Input: part model. Units: mm. Frame: model coordinates. A direction names the side the tool comes from. Give positions to 0.01 mm unless a question says otherwise; leave off trailing zeros. Loops run counter-clockwise (first coordinate to the right, second up) from the corner with the lowest first, then second, coordinate; pieces in that order, holes last. Notation, with made-up numbers: (51, 0) -> (63, 0) arc R7 cw to (63, 9) -> close; hole circle Ø5 at (18, 33). An arc over 180 degrees is marked (long way). One line per question, with ' | ' between items.
Autodesk Inventor part; units mm, degrees
ref_plane "YZ Plane" through (0, 0, 0) normal (1, 0, 0) x (0, 1, 0)
ref_plane "XZ Plane" through (0, 0, 0) normal (0, 1, 0) x (-1, 0, 0)
ref_plane "XY Plane" through (0, 0, 0) normal (0, 0, 1) x (1, 0, 0)
sketch "Sketch1" plane through (0, 0, 0) normal (1, 0, 0) x (0, 1, 0)
  arc A0 (-67.3092, -213.4776) -> (57.9334, -216.2104) centre (0, 0) ccw
  arc A1 (-69.6961, -221.0477) -> (59.9878, -223.8775) centre (0, 0) ccw construction
  line L0 (0, 0) -> (-69.6961, -221.0477) construction
  line L1 (0, 0) -> (59.9878, -223.8775) construction
  line L2 (59.9878, -223.8775) -> (57.9334, -216.2104) construction
  line L3 (0, -287.3347) -> (0, 47.8891) construction
  arc A2 (-69.6961, -227.6971) -> (59.9878, -230.4452) centre (0, 0) ccw
  arc A3 (-68.5027, -217.2627) -> (58.9606, -220.0439) centre (0, 0) ccw construction
  arc A4 (-68.5027, -217.2627) -> (-53.1803, -221.5119) centre (0, 0) ccw
  line L4 (-53.1803, -221.5119) -> (0, 0) construction
  arc A5 (-35.1466, -206.5815) -> (27.3518, -207.7573) centre (0, 0) ccw construction
  line L5 (0, 0) -> (27.3518, -207.7573) construction
  line L6 (0, 0) -> (209.55, 0) construction
  circle A6 centre (27.3518, -207.7573) radius 15.5575
  circle A7 centre (-35.1466, -206.5815) radius 15.5575
  line L7 (59.9878, -230.4452) -> (57.9334, -216.2104)
  line L8 (-69.6961, -227.6971) -> (-67.3092, -213.4776)
  point P0 (-26.7758, -226.2272)
  point P1 (0, -227.8063)
  point P2 (26.7758, -226.2272)
  point P3 (53.1803, -221.5119)
  point P4 (35.5128, -221.0024)
  point P5 (22.8969, -222.6633)
  point P6 (-31.2556, -221.6446)
  point P7 (-43.8, -219.5103)
  dimension "d0" = 223.8375
  dimension "d1" = 231.775
  dimension "d2" = 32.5
  dimension "d3" = 15
  dimension "d4" = 238.125
  dimension "d5" = 4
  dimension "d8" = 27
  dimension "d19" = 209.55
  dimension "d20" = 82.5
  dimension "d21" = 62.5094
  dimension "d22" = 31.115
  dimension "d23" = 31.115
extrude "Extrusion1" add sketch "Sketch1" along normal blind 2.54 contours A0 A7 A6 L7 A2 L8
hole "Hole1" at (0, -53.1803, -221.5119) at (0, -26.7758, -226.2272) at (0, 0, -227.8063) at (0, 26.7758, -226.2272) at (0, 53.1803, -221.5119) direction (1, 0, 0) diameter 3.2004 end through all
fillet "Fillet1" radius 3.175 8 edges at (1.27, 57.9334, -216.2104) (1.27, 59.9878, -230.4452) (1.27, 35.5128, -221.0024) (1.27, 22.8969, -222.6633) (1.27, -31.2556, -221.6446) (1.27, -43.8, -219.5103) (1.27, -67.3092, -213.4776) (1.27, -69.6961, -227.6971)
properties part number "3DPRINT,HOOD,ALIGNMENT,PLATES" material "Nylon 6/6"
1. Pin query (flat end, axial travel): P1, Ø2.5, axis at y = -26.78, z = -226.23, coming from the -X side; P2, Ø1.5, axis at x = 1.5, z = -219.5, coming from the +Y side. Return the tip coordinate at first contact, or that it passes through.
Determined:
P1: passes through | P2: stops at y = 58.52
2. Ray query, line 1 along Z through (x, y) = (0.85, 0) (1 decimal); line 2 along Z through (x, y) = (1.45, 25.5); line 3 along Z through (x, y) = (0.55, 34.5). Return the intervals inside material, ascending. Write a range as from..to.
Determined:
line 1: z = -238.1..-229.4, -226.2..-223.8 | line 2: z = -236.76..-227.19, -225.26..-223.2 | line 3: z = -235.61..-221.58
3. Section query B-B (x = 1.7). Count the separate pieces of the cut face and the enclosed holes in it, then the cut area to 3 significant figures.
Determined:
separate pieces: 1 | enclosed holes: 5 | area: 1,770 mm2
4. Section query D-D (y = -42). Output: boundary loops of the cut face in (x, z), then the cut area to 3 significant figures.
Determined:
outline: (0, -234.39) -> (2.54, -234.39) -> (2.54, -220.55) -> (0, -220.55) -> close | area: 35.2 mm2
5. Section query A-A (y = 0). Output: boundary loops of the cut face in (x, z) (1 decimal), then the cut area to 3 significant figures.
Determined:
outline: (0, -238.1) -> (2.5, -238.1) -> (2.5, -229.4) -> (0, -229.4) -> close; (0, -226.2) -> (2.5, -226.2) -> (2.5, -223.8) -> (0, -223.8) -> close | area: 28.2 mm2
6. Reachability of faces 1 (the flat face through (0, -6, -229)), 2 (the cylindrical face through (1.25, 45.48, -219.17)) from +Z, -Z, +X, -X, +Y, -Y: full face, straight path, thin tool, end or side. Return the list, or none.
Determined:
face 1: +Z, -Z, -X, +Y, -Y | face 2: +Z, +X, -X
7. Pull-direction query (Y, two-part tool) for faces 3 (the cylindrical face through (1.288, -66.425, -214.86)), 4 (the cylindrical face through (1.288, -68.809, -227.118)), 5 (the cylindrical face through (1.288, 52.7, -219.986)), 6 (the flat face through (1.252, 59.018, -223.724)); classes: pulls with the +Y half, pulls with the -Y half, needs draft (parallel to the pull), parting line crosses it, or undercut.
Determined:
face 3: parting line crosses it | face 4: pulls with the -Y half | face 5: undercut | face 6: pulls with the +Y half
